Source: three-view drawing plus pictorial views. Frame: mm from the lowest corner of the part. A direction names the side the tool comes from. Round coordinates to 2 decimals unless told otherwise and drop trailing zeros. Order: outer loops, then holes, each group sorted by start corner. A loop starts at its lowest first (then second) coordinate and runs counter-clockwise, first axis right, second up. Notation, with made-up numbers: (-36, -23.5) -> (-20, -23.5) arc R29 cw to (-20, 2.5) -> close; hole circle Ø6 at (17.25, -6.5). An arc over 180 degrees is marked (long way). Use a Markdown table: item, result.
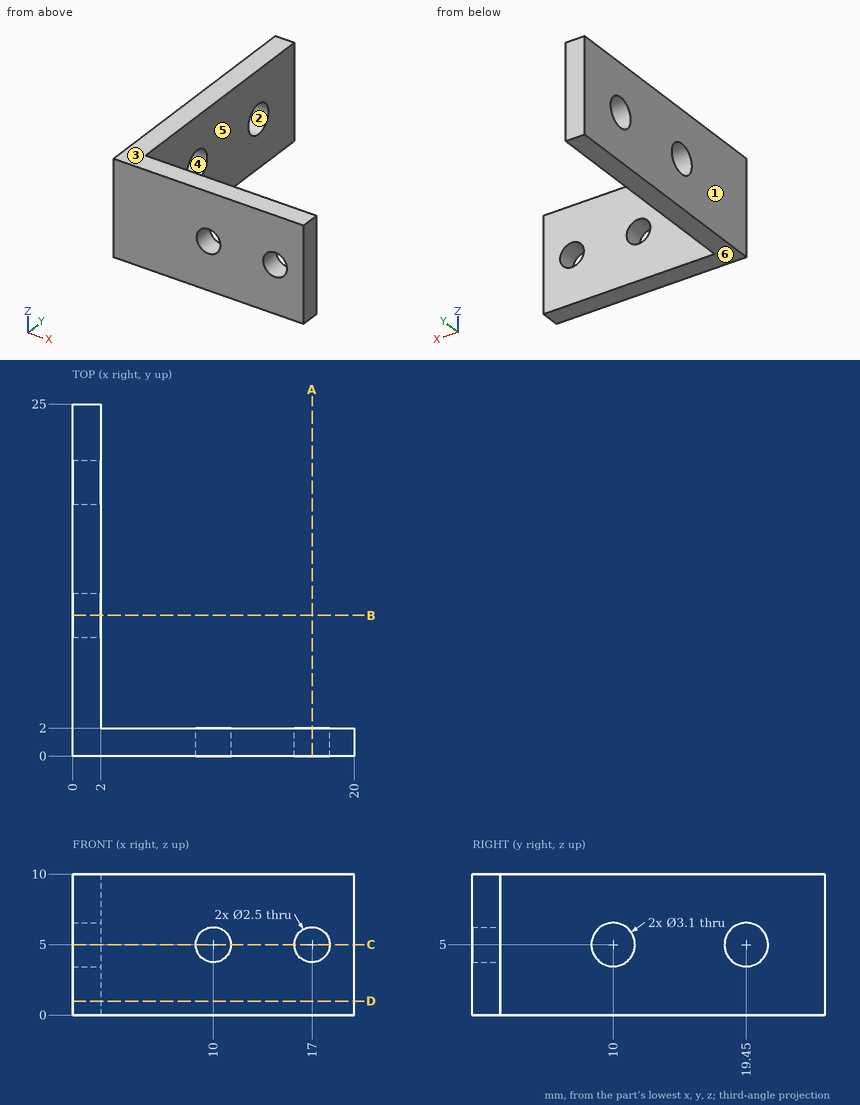
1) Cut plane A-A on x = 17. Return loops of the section in (y, z).
Results found:
| item | result |
|---|---|
| outline | (0, 0) -> (2, 0) -> (2, 3.75) -> (0, 3.75) -> close; (0, 6.25) -> (2, 6.25) -> (2, 10) -> (0, 10) -> close |
2) Cut plane D-D on z = 1. Return loops of the section in (x, y).
Results found:
| item | result |
|---|---|
| outline | (0, 0) -> (20, 0) -> (20, 2) -> (2, 2) -> (2, 25) -> (0, 25) -> close |
3) Cut plane C-C on z = 5. Return loops of the section in (x, y), and give its area (3 significant figures).
Results found:
| item | result |
|---|---|
| outline | (0, 0) -> (8.75, 0) -> (8.75, 2) -> (2, 2) -> (2, 8.45) -> (0, 8.45) -> close; (0, 11.55) -> (2, 11.55) -> (2, 17.9) -> (0, 17.9) -> close; (0, 21) -> (2, 21) -> (2, 25) -> (0, 25) -> close; (11.25, 0) -> (15.75, 0) -> (15.75, 2) -> (11.25, 2) -> close; (18.25, 0) -> (20, 0) -> (20, 2) -> (18.25, 2) -> close |
| area | 63.6 mm² |
4) Pin query (flat end, axial travel): pin 1 Ø6 at (y, z) = (8, 6) entering from -X; pin 2 Ø3 at (x, z) = (17, 5) entering from +Y; pin 3 Ø1.5 at (y, z) = (3, 4.5) entering from +X. Return the tip coordinate at first contact, or that it passes through.
Results found:
| item | result |
|---|---|
| pin 1 | stops at x = 0 |
| pin 2 | stops at y = 2 |
| pin 3 | stops at x = 2 |
5) Set-up query: the marked faces 5 and 6. Return all of +Z, -Z, +X, -X, +Y, -Y with unobstructed straight access to the full face (end or side cutting, diameter ignored); none if empty.
Results found:
| item | result |
|---|---|
| face 5 | +Z, -Z, +X, +Y |
| face 6 | -Z, +X, -X, +Y, -Y |
6) Pull-direction query (Z, two-part tool) for the marked faces 1, 2, 3 and 4; classes: +Z half, -Z half, draft (parallel to the pull), parting line (faces both ways), or undercut.
Results found:
| item | result |
|---|---|
| face 1 | draft |
| face 2 | undercut |
| face 3 | +Z half |
| face 4 | undercut |
7) Cut plane B-B on y = 10. Return loops of the section in (x, z).
Results found:
| item | result |
|---|---|
| outline | (0, 0) -> (2, 0) -> (2, 3.45) -> (0, 3.45) -> close; (0, 6.55) -> (2, 6.55) -> (2, 10) -> (0, 10) -> close |
8) Line query: L1, parallel to X at y = 1.3, z = 5; L2, parallel to Y at x = 1.2, z = 5; L3, parallel to Z at x = 17, y = 1.55. Output: solid intervals per line, ascending. Write a range as [from, to].
Results found:
| item | result |
|---|---|
| L1 | x = [0, 8.75], [11.25, 15.75], [18.25, 20] |
| L2 | y = [0, 8.45], [11.55, 17.9], [21, 25] |
| L3 | z = [0, 3.75], [6.25, 10] |
